Geometry check sheet. Reference: the model listing, model coordinates, mm. Face numbers are marked on the shaded views. A direction names the side the tool comes from. Coordinates: 2 decimals unless noted, no trailing zeros. Loops run counter-clockwise (first coordinate to the right, second up) from the corner with the lowest first, then second, coordinate; pieces in that order, holes last. Notation, with made-up numbers: (-32, -1.5) -> (19, -1.5) arc R19 ccw to (19, 22.5) -> close; hole circle Ø5 at (4.25, 30). An arc over 180 degrees is marked (long way). Answer as a JSON object with one key per item and string values.
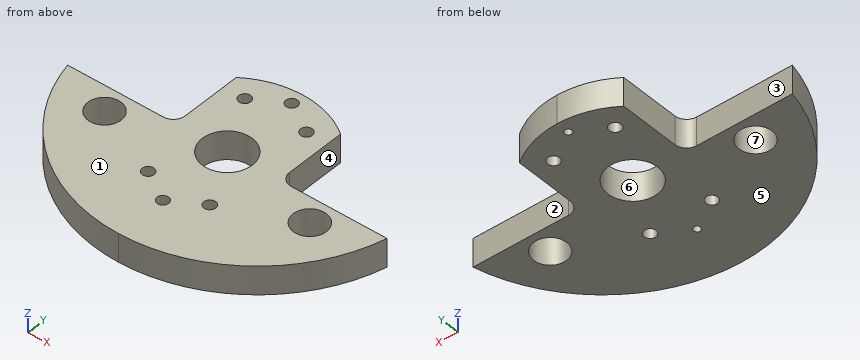
from build123d import *

# Parameters (mm, degrees)
F2_R           = 2.5
F2_R_2         = 10.5
F3_DEPTH       = 12
F4_D           = 3
F4_CBORE_D     = 4.9
F4_CBORE_DEPTH = 7
F5_D           = 14


with BuildPart() as f3:
    # F2 (on offset) → F3 (new body)
    with BuildSketch(Plane.XY.offset(-19)):
        with BuildLine():
            Line((-27, 0), (-67.349833, 0))
            ThreePointArc((-67.349833, 0), (-43.162484, -38.833075), (0, -54))
            ThreePointArc((0, -54), (43.162484, -38.833075), (67.349833, 0))
            Line((67.349833, 0), (27, 0))
            ThreePointArc((27, 0), (23.464466, 1.464466), (22, 5))
            Line((22, 5), (22, 30.368569))
            ThreePointArc((22, 30.368569), (11.563491, 35.672618), (0, 37.5))
            ThreePointArc((0, 37.5), (-11.563491, 35.672618), (-22, 30.368569))
            Line((-22, 30.368569), (-22, 5))
            ThreePointArc((-22, 5), (-23.464466, 1.464466), (-27, 0))
        make_face()
        with Locations((-13, -24)):
            Circle(F2_R, mode=Mode.SUBTRACT)
        with Locations((13, -24)):
            Circle(F2_R, mode=Mode.SUBTRACT)
        with Locations((-13, 24)):
            Circle(F2_R, mode=Mode.SUBTRACT)
        Circle(F2_R_2, mode=Mode.SUBTRACT)
        with Locations((13, 24)):
            Circle(F2_R, mode=Mode.SUBTRACT)
    extrude(amount=-F3_DEPTH)

    # F4 (through all)
    with Locations(Plane.XY.offset(-19)):
        with Locations((0, 32), (0, -32)):
            CounterBoreHole(F4_D / 2, F4_CBORE_D / 2, F4_CBORE_DEPTH)

    # F5 (through all)
    with Locations(Plane.XY):
        with Locations((-43.30127, -10), (43.30127, -10)):
            Hole(F5_D / 2)


solid = f3.part
1. Section check A-A, the plane y = 3.5. Record the boundary of the cut face in (x, z).
Evaluation:
{"outline": "(-22.23, -31) -> (-9.9, -31) -> (-9.9, -19) -> (-22.23, -19) -> close; (9.9, -31) -> (22.23, -31) -> (22.23, -19) -> (9.9, -19) -> close"}
2. Section check C-C, the plane x = 40. Record the boundary of the cut face in (y, z), then the cut area to 3 significant figures.
Evaluation:
{"outline": "(-41.22, -31) -> (-16.17, -31) -> (-16.17, -19) -> (-41.22, -19) -> close; (-3.83, -31) -> (0, -31) -> (0, -19) -> (-3.83, -19) -> close", "area": "347 mm^2"}
3. Thickness scan on probe 1 along Y at (x, z) = (0, -25); probe 2 along Y at (x, z) = (0, -28.4); probe 3 along X at (y, z) = (-13, -24.5). Record the ranges inside material, lowest first. Write a range as from..to.
Evaluation:
{"probe 1": "y = -54..-34.45, -29.55..-10.5, 10.5..29.55, 34.45..37.5", "probe 2": "y = -54..-33.5, -30.5..-10.5, 10.5..30.5, 33.5..37.5", "probe 3": "x = -63.06..-49.63, -36.98..36.98, 49.63..63.06"}
4. Section check B-B, the plane z = -23. State how many separate pieces and enclosed holes the cut face has, then the cut area to 3 significant figures.
Evaluation:
{"separate pieces": "1", "enclosed holes": "9", "area": "6,210 mm^2"}
5. Depth check by flat-ended pin: P1, Ø6, axis at x = 26.5, z = -27, coming from the +Y side; P2, Ø1, axis at y = 25.5, z = -24.5, coming from the +X side; P3, Ø10, axis at x = 44.5, y = 1.5, coming from the -Z side; P4, Ø3.5, axis at y = 22.5, z = -25.5, coming from the -X side. Enter the tip coordinate at first touch or a pass-through.
Evaluation:
{"P1": "stops at y = 1.43", "P2": "stops at x = 22", "P3": "stops at z = -31", "P4": "stops at x = -22"}
6. Section check D-D, the plane x = 12. Record the boundary of the cut face in (y, z).
Evaluation:
{"outline": "(-52.95, -31) -> (-26.29, -31) -> (-26.29, -19) -> (-52.95, -19) -> close; (-21.71, -31) -> (21.71, -31) -> (21.71, -19) -> (-21.71, -19) -> close; (26.29, -31) -> (35.53, -31) -> (35.53, -19) -> (26.29, -19) -> close"}
7. Mould release check, pull along X, two halves, no side actions. Record for the marked faces 4, 5, 6 and 7: released by +X, released by -X, zero draft, split by the parting line, or undercut.
Evaluation:
{"face 4": "released by +X", "face 5": "zero draft", "face 6": "undercut", "face 7": "undercut"}
8. Tool access check on the marked faces 1, 2 and 3. Record the directions out of +Z, -Z, +X, -X, +Y, -Y that give a thin tool (end or side, any length) a straight path to the whole face; none if there is none.
Evaluation:
{"face 1": "+Z, +X, -X, +Y, -Y", "face 2": "+Z, -Z, +X, +Y", "face 3": "+Z, -Z, -X, +Y"}
